Drawing for the job (mm, zero at the part's lowest x, y, z). A direction names the side the tool comes from. Give positions to 0.01 mm unless a question says otherwise; leave off trailing zeros. Order: outer loops, then holes, each group sorted by start corner. A loop starts at its lowest first (then second) coordinate and runs counter-clockwise, first axis right, second up. Notation, with made-up numbers: (48.25, 17.5) - (77.25, 17.5) arc R29 cw to (77.25, 54.5) - close; hole circle Ø11 at (-10, -17). An arc over 180 degrees is marked (long way). Use a Markdown table: item, result.
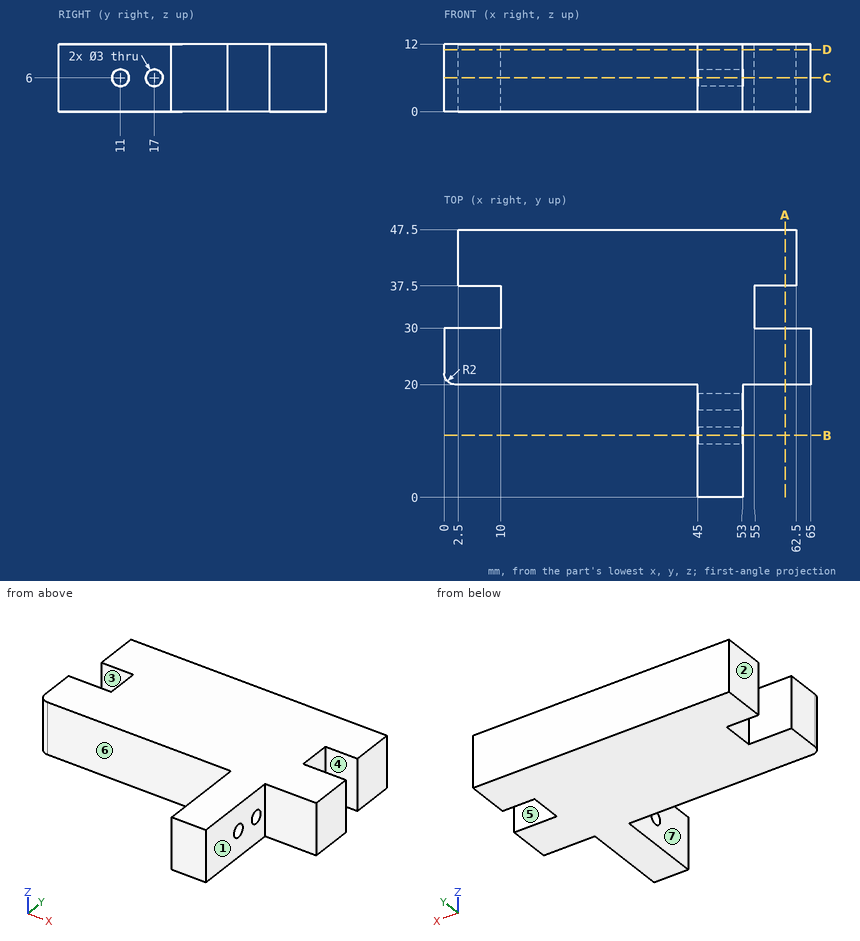
1) Slice it at D-D (z = 11). Write the cut outline in (x, y), and give its area (3 significant figures).
Computed:
| item | result |
|---|---|
| outline | (0, 22) arc R2 ccw to (2, 20) - (45, 20) - (45, 0) - (53, 0) - (53, 20) - (65, 20) - (65, 30) - (55, 30) - (55, 37.5) - (62.5, 37.5) - (62.5, 47.5) - (2.5, 47.5) - (2.5, 37.5) - (10, 37.5) - (10, 30) - (0, 30) - close |
| area | 1,750 mm² |
2) Slice it at A-A (x = 60.5). Write the cut outline in (y, z), and give its area (3 significant figures).
Computed:
| item | result |
|---|---|
| outline | (20, 0) - (30, 0) - (30, 12) - (20, 12) - close; (37.5, 0) - (47.5, 0) - (47.5, 12) - (37.5, 12) - close |
| area | 240 mm² |
3) Wall check: line 1 (Y direction, x = 50, z = 6); line 2 (Z direction, x = 51.5, y = 17); line 3 (Y direction, x = 47, z = 7.25). Give the ranges that are in metal, low to high. Write a range as from..to.
Computed:
| item | result |
|---|---|
| line 1 | y = 0..9.5, 12.5..15.5, 18.5..47.5 |
| line 2 | z = 0..4.5, 7.5..12 |
| line 3 | y = 0..10.17, 11.83..16.17, 17.83..47.5 |
4) Pin check, flat tips, straight feed: P1, Ø6, axis at y = 9.5, z = 7, coming from the -X side; P2, Ø5, axis at x = 28.5, z = 9, coming from the -Y side; P3, Ø5, axis at y = 41.5, z = 7.5, coming from the -X side. Stop position of each tip, or through.
Computed:
| item | result |
|---|---|
| P1 | stops at x = 45 |
| P2 | stops at y = 20 |
| P3 | stops at x = 2.5 |
5) Tool access for the marked faces 1, 2, 3 and 4: list every direction of +Z, -Z, +X, -X, +Y, -Y with a clear straight run to the whole face (end or side of a thin tool).
Computed:
| item | result |
|---|---|
| face 1 | +Z, -Z, +X, -Y |
| face 2 | +Z, -Z, -X, +Y |
| face 3 | +Z, -Z, -X |
| face 4 | +Z, -Z, +X |
6) Two-plate mould, pull along Y, no slides. Class the marked faces 5, 6 and 7: +Y half, -Y half, draft (parallel to the pull), parting line (faces both ways), or undercut.
Computed:
| item | result |
|---|---|
| face 5 | undercut |
| face 6 | -Y half |
| face 7 | draft |
7) Slice it at B-B (y = 11). Write the cut outline in (x, z).
Computed:
| item | result |
|---|---|
| outline | (45, 0) - (53, 0) - (53, 4.5) - (45, 4.5) - close; (45, 7.5) - (53, 7.5) - (53, 12) - (45, 12) - close |
8) Slice it at C-C (z = 6). Write the cut outline in (x, y).
Computed:
| item | result |
|---|---|
| outline | (0, 22) arc R2 ccw to (2, 20) - (45, 20) - (45, 18.5) - (53, 18.5) - (53, 20) - (65, 20) - (65, 30) - (55, 30) - (55, 37.5) - (62.5, 37.5) - (62.5, 47.5) - (2.5, 47.5) - (2.5, 37.5) - (10, 37.5) - (10, 30) - (0, 30) - close; (45, 0) - (53, 0) - (53, 9.5) - (45, 9.5) - close; (45, 12.5) - (53, 12.5) - (53, 15.5) - (45, 15.5) - close |
